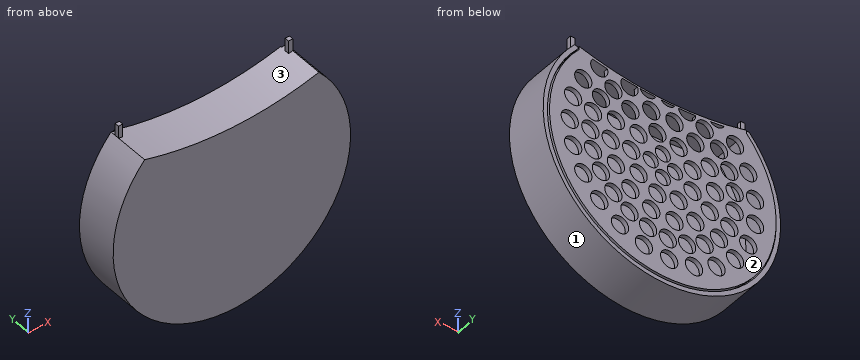
from build123d import *

# Parameters (mm, degrees)
SKETCH1_R           = 69.85
BODY_DEPTH          = 25.4
SHELL1_T            = -2.54
SKETCH3_R           = 66.675
PLATE_DEPTH         = 2.54
SKETCH5_R           = 5.08
CUT_EXTRUDE2_DEPTH  = 2.54
CIRPATTERN1_COUNT   = 23
SKETCH6_R           = 5.08
CUT_EXTRUDE3_DEPTH  = 2.54
CIRPATTERN2_COUNT   = 14
SKETCH7_R           = 5.08
CUT_EXTRUDE4_DEPTH  = 2.54
CIRPATTERN3_COUNT   = 9
SKETCH8_R           = 4.445
CUT_EXTRUDE5_DEPTH  = 2.54
CIRPATTERN4_COUNT   = 4
BOSS_EXTRUDE1_DEPTH = 25.4
CIRCLE_CUT_DEPTH    = 63.5
CUT_EXTRUDE6_DEPTH  = 63.5
SKETCH12_W          = 2.54
SKETCH12_H          = 2.54
CONNECTORS_DEPTH    = 7.62


with BuildPart() as part:
    # Sketch1 → Body (new body)
    with BuildSketch(Plane(origin=(0, 0, 0), x_dir=(1, 0, 0), z_dir=(0, 1, 0))):
        with Locations(Location((0, 0, 0), (0, 0, 270))):
            Circle(SKETCH1_R)
    extrude(amount=BODY_DEPTH)

    # Shell1
    shell1_openings = [part.faces().sort_by_distance(p)[0] for p in [
        (0, 25.4, 0),
    ]]
    offset(amount=SHELL1_T, openings=shell1_openings, kind=Kind.INTERSECTION)



with BuildPart() as body_2:
    # Sketch3 → plate (new body)
    with BuildSketch(Plane(origin=(0, 26.162, 0), x_dir=(1, 0, 0), z_dir=(0, 1, 0))):
        with Locations(Location((0, 0, 0), (0, 0, 270))):
            Circle(SKETCH3_R)
    extrude(amount=-PLATE_DEPTH)

    # Sketch5 → Cut-Extrude2 (cut)
    with BuildSketch(Plane(origin=(0, 26.162, 0), x_dir=(1, 0, 0), z_dir=(0, 1, 0))):
        with Locations(Location((54.789530839, 0, 0), (0, 0, 270))):
            Circle(SKETCH5_R)
        with Locations(Location((42.654572856, 0, 0), (0, 0, 270))):
            Circle(SKETCH5_R)
    cut_extrude2 = extrude(amount=-CUT_EXTRUDE2_DEPTH, mode=Mode.SUBTRACT)

    # CirPattern1: Cut-Extrude2 ×23 about axis
    cirpattern1_axis = Axis((0, 0, 0), (0, 1, 0))
    for i in range(1, CIRPATTERN1_COUNT):
        add(cut_extrude2.rotate(cirpattern1_axis, i * 360 / CIRPATTERN1_COUNT), mode=Mode.SUBTRACT)

    # Sketch6 → Cut-Extrude3 (cut)
    with BuildSketch(Plane(origin=(0, 26.162, 0), x_dir=(1, 0, 0), z_dir=(0, 1, 0))):
        with Locations(Location((30.667157657, 0, 0), (0, 0, 270))):
            Circle(SKETCH6_R)
    cut_extrude3 = extrude(amount=-CUT_EXTRUDE3_DEPTH, mode=Mode.SUBTRACT)

    # CirPattern2: Cut-Extrude3 ×14 about axis
    cirpattern2_axis = Axis((0, 0, 0), (0, 1, 0))
    for i in range(1, CIRPATTERN2_COUNT):
        add(cut_extrude3.rotate(cirpattern2_axis, i * 360 / CIRPATTERN2_COUNT), mode=Mode.SUBTRACT)

    # Sketch7 → Cut-Extrude4 (cut)
    with BuildSketch(Plane(origin=(0, 26.162, 0), x_dir=(1, 0, 0), z_dir=(0, 1, 0))):
        with Locations(Location((18.602614166, 0, 0), (0, 0, 270))):
            Circle(SKETCH7_R)
    cut_extrude4 = extrude(amount=-CUT_EXTRUDE4_DEPTH, mode=Mode.SUBTRACT)

    # CirPattern3: Cut-Extrude4 ×9 about axis
    cirpattern3_axis = Axis((0, 0, 0), (0, 1, 0))
    for i in range(1, CIRPATTERN3_COUNT):
        add(cut_extrude4.rotate(cirpattern3_axis, i * 360 / CIRPATTERN3_COUNT), mode=Mode.SUBTRACT)

    # Sketch8 → Cut-Extrude5 (cut)
    with BuildSketch(Plane(origin=(0, 26.162, 0), x_dir=(1, 0, 0), z_dir=(0, 1, 0))):
        with Locations(Location((7.129637739, 0, 0), (0, 0, 270))):
            Circle(SKETCH8_R)
    cut_extrude5 = extrude(amount=-CUT_EXTRUDE5_DEPTH, mode=Mode.SUBTRACT)

    # CirPattern4: Cut-Extrude5 ×4 about axis
    cirpattern4_axis = Axis((0, 0, 0), (0, 1, 0))
    for i in range(1, CIRPATTERN4_COUNT):
        add(cut_extrude5.rotate(cirpattern4_axis, i * 360 / CIRPATTERN4_COUNT), mode=Mode.SUBTRACT)


with BuildPart() as part_1:
    add(part.part)

    add(body_2.part)  # Boss-Extrude1 merges body 2
    # Sketch13 → Boss-Extrude1 (add, symmetric)
    with BuildSketch(Plane(origin=(0, 25.4, 0), x_dir=(1, 0, 0), z_dir=(0, 1, 0))):
        with BuildLine():
            Line((49.237524928, -86.868), (-49.237524928, -86.868))
            Line((-49.237524928, -86.868), (-49.237524928, -44.958))
            ThreePointArc((-49.237524928, -44.958), (0, -39.388206386), (49.237524928, -44.958))
            Line((49.237524928, -44.958), (49.237524928, -86.868))
        make_face()
    extrude(amount=BOSS_EXTRUDE1_DEPTH, both=True)

    # Sketch9 → circle cut (cut, symmetric)
    with BuildSketch(Plane(origin=(0, 0, 0), x_dir=(1, 0, 0), z_dir=(0, 1, 0))):
        with BuildLine():
            Line((69.85, -86.892577), (-69.85, -86.892577))
            Line((-69.85, -86.892577), (-69.85, -53.720370546))
            ThreePointArc((-69.85, -53.720370546), (0, -40.286677853), (69.85, -53.720370546))
            Line((69.85, -53.720370546), (69.85, -86.892577))
        make_face()
    extrude(amount=CIRCLE_CUT_DEPTH, both=True, mode=Mode.SUBTRACT)

    # Sketch14 → Cut-Extrude6 (cut, symmetric)
    with BuildSketch(Plane(origin=(0, 0, 0), x_dir=(0, 0, -1), z_dir=(1, 0, 0))):
        Polygon((-23.267075151, 26.162), (-48.667075151, 26.162), (-48.667075151, 52.593802599), (-39.427592482, 52.593802599), align=None)
    extrude(amount=CUT_EXTRUDE6_DEPTH, both=True, mode=Mode.SUBTRACT)

    # Sketch12 → connectors (add)
    with BuildSketch(Plane.XY.offset(46.99)):
        with Locations((-50.027909309, 21.082)):
            Rectangle(SKETCH12_W, SKETCH12_H)
        with Locations((50.027909309, 21.082)):
            Rectangle(SKETCH12_W, SKETCH12_H)
    extrude(amount=CONNECTORS_DEPTH)


solid = part_1.part
Source: CAD feature listing. Evaluate the final solid. Frame: model axes, mm. Face numbers are marked on the shaded views. Give positions to 0.01 mm unless a question says otherwise; leave off trailing zeros. Order: outer loops, then holes, each group sorted by start corner. A loop starts at its lowest first (then second) coordinate and runs counter-clockwise, first axis right, second up. Notation, with made-up numbers: (50.25, 67) -> (81.25, 67) arc R21 ccw to (81.25, 79) -> close; hole circle Ø5 at (54, -30.5). An arc over 180 degrees is marked (long way). Write item = value, one per line.
Item 1: Mould query, pull axis X, two halves, no side actions, for the marked faces 1, 2 and 3. Classes: +X half, -X half, draft (parallel to the pull), parting line (faces both ways), or undercut.
Check result:
face_1 = parting line
face_2 = draft
face_3 = undercut
Item 2: Section query B-B (z = -15). State how many separate pieces and enclosed holes the cut face has, then the cut area to 3 significant figures.
Check result:
separate_pieces = 10
enclosed_holes = 0
area = 613 mm²
Item 3: Contact query for flat-ended pins moving along their axis: pin 1 (1.5 mm diameter, centred on x = 42, y = 13.5, fed in from -Z); pin 2 (8 mm diameter, centred on x = 46.81, z = -28.47, fed in from +Y); pin 3 (4 mm diameter, centred on x = 15.5, y = 17.5, fed in from -Z). Output: stop coordinate, or through.
Check result:
pin_1 = -56.37
pin_2 = 2.54
pin_3 = -68.53
Item 4: Ray query, probe 1 along Y at (x, z) = (56, 31.5); probe 2 along Z at (x, y) = (1.5, 8.25); probe 3 along X at (y, z) = (17.75, 35). Return the intervals inside material, ascending.
Check result:
probe_1 = 0 to 2.54, 23.62 to 26.16
probe_2 = -69.83 to -67.29, 39.39 to 40.29
probe_3 = -60.45 to -57.49, 57.49 to 60.45
Item 5: Section query A-A (y = 9.25). Output: boundary loops of the cut face in (x, z).
Check result:
outline = (-51.3, 47.41) arc R69.85 ccw (long way) to (51.3, 47.41) arc R188.31 cw to start; hole (-49.24, 44.96) -> (-49.24, 45.89) arc R67.31 ccw (long way) to (49.24, 45.89) -> (49.24, 44.96) arc R220.42 cw to start
